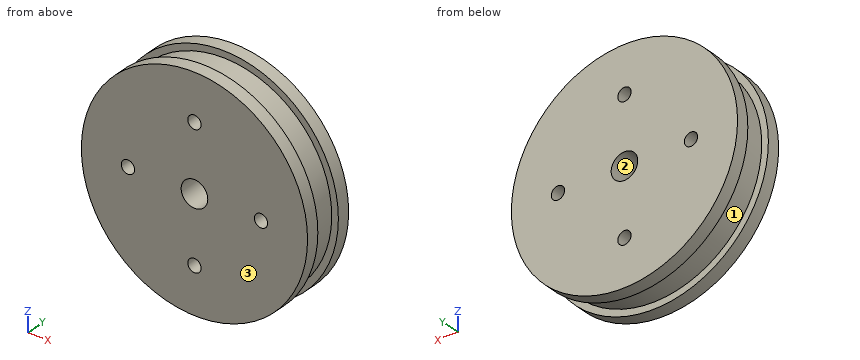
from build123d import *

# Parameters (mm, degrees)
F0_R     = 53.975
F1_DEPTH = 6.35
F2_R     = 50.8
F3_DEPTH = 12.7
F4_R     = 53.975
F5_DEPTH = 6.35
F7_D     = 6.35
F8_R     = 6.35
F9_DEPTH = 25.401


with BuildPart() as f1:
    # F0 (on Front) → F1 (new body)
    with BuildSketch(Plane.XZ):
        Circle(F0_R)
    extrude(amount=F1_DEPTH)

    # F2 (on face) → F3 (join)
    with BuildSketch(Plane.XZ.offset(6.35)):
        Circle(F2_R)
    extrude(amount=F3_DEPTH)

    # F4 (on face) → F5 (join)
    with BuildSketch(Plane.XZ.offset(19.05)):
        Circle(F4_R)
    extrude(amount=F5_DEPTH)

    # F7 (through all)
    with Locations(Plane.XZ.offset(25.4)):
        with Locations((0, 31.75), (31.75, 0), (0, -31.75), (-31.75, 0)):
            Hole(F7_D / 2)

    # F8 (on face) → F9 (cut, through all)
    with BuildSketch(Plane.XZ.offset(25.4)):
        Circle(F8_R)
    extrude(amount=-F9_DEPTH, mode=Mode.SUBTRACT)


solid = f1.part
Input: part model. Units: mm. Frame: model coordinates. Face numbers are marked on the shaded views. Coordinates: 2 decimals unless noted, no trailing zeros. Loops run counter-clockwise (first coordinate to the right, second up) from the corner with the lowest first, then second, coordinate; pieces in that order, holes last. Notation, with made-up numbers: (16.5, 64.5) -> (67.5, 64.5) arc R29 cw to (67.5, 96.5) -> close; hole circle Ø5 at (31, 9.25). An arc over 180 degrees is marked (long way). Write item = value, one per line. Start each with the question number.
Item 1: Mould query, pull axis Z, two halves, no side actions, for the marked faces 1, 2 and 3. Classes: pulls with the +Z half, pulls with the -Z half, needs draft (parallel to the pull), parting line crosses it, or undercut.
Item 2: Cut plane A-A, the plane z = 0. Return loops of the section in (x, y) (3 decimals).
Item 3: Material intervals for line 1 (Z direction, x = 0, y = -7) (3 decimals); line 2 (X direction, y = -17, z = 1.5); line 3 (Y direction, x = -48, z = -22.5), sorted ascending.
Item 4: Cut plane B-B, the plane x = 33.5. Return loops of the section in (y, z).
Item 5: First-contact query: P1, Ø12, axis at x = -10.5, y = -22, coming from the +Z side; P2, Ø2, axis at x = 8.5, z = 15, coming from the +Y side; P3, Ø2, axis at x = -13.5, y = -12.5, coming from the +Z side; P4, Ø3, axis at x = -9.5, y = -20, coming from the +Z side. Flat tips, straight axial feed; report the tip coordinate or a pass-through.
Item 6: Cut plane C-C, the plane z = 31.75. Return loops of the section in (x, y) (3 decimals), plus the area to 3 significant figures.
Item 7: Cut plane D-D, the plane y = -12.5. Return loops of the section in (x, z) (3 decimals).
Ans:
q1.face_1 = parting line crosses it
q1.face_2 = undercut
q1.face_3 = needs draft
q2.outline = (-53.975, -25.4) -> (-34.925, -25.4) -> (-34.925, 0) -> (-53.975, 0) -> (-53.975, -6.35) -> (-50.8, -6.35) -> (-50.8, -19.05) -> (-53.975, -19.05) -> close; (-28.575, -25.4) -> (-6.35, -25.4) -> (-6.35, 0) -> (-28.575, 0) -> close; (6.35, -25.4) -> (28.575, -25.4) -> (28.575, 0) -> (6.35, 0) -> close; (34.925, -25.4) -> (53.975, -25.4) -> (53.975, -19.05) -> (50.8, -19.05) -> (50.8, -6.35) -> (53.975, -6.35) -> (53.975, 0) -> (34.925, 0) -> close
q3.line_1 = -50.8 to -34.925, -28.575 to -6.35, 6.35 to 28.575, 34.925 to 50.8
q3.line_2 = -50.78 to -34.55, -28.95 to -6.17, 6.17 to 28.95, 34.55 to 50.78
q3.line_3 = -25.4 to -19.05, -6.35 to 0
q4.outline = (-25.4, -42.32) -> (-19.05, -42.32) -> (-19.05, -38.19) -> (-6.35, -38.19) -> (-6.35, -42.32) -> (0, -42.32) -> (0, -2.65) -> (-25.4, -2.65) -> close; (-25.4, 2.65) -> (0, 2.65) -> (0, 42.32) -> (-6.35, 42.32) -> (-6.35, 38.19) -> (-19.05, 38.19) -> (-19.05, 42.32) -> (-25.4, 42.32) -> close
q5.P1 = 53.79
q5.P2 = 0
q5.P3 = 49.24
q5.P4 = 53.38
q6.outline = (-43.649, -25.4) -> (-3.175, -25.4) -> (-3.175, 0) -> (-43.649, 0) -> (-43.649, -6.35) -> (-39.656, -6.35) -> (-39.656, -19.05) -> (-43.649, -19.05) -> close; (3.175, -25.4) -> (43.649, -25.4) -> (43.649, -19.05) -> (39.656, -19.05) -> (39.656, -6.35) -> (43.649, -6.35) -> (43.649, 0) -> (3.175, 0) -> close
q6.area = 1,950 mm²
q7.outline = circle Ø101.6 at (0, 0); hole circle Ø6.35 at (-31.75, 0); hole circle Ø12.7 at (0, 0); hole circle Ø6.35 at (0, -31.75); hole circle Ø6.35 at (0, 31.75); hole circle Ø6.35 at (31.75, 0)
